Part model, mm, in its own coordinate system. A direction names the side the tool comes from. Give positions to 0.01 mm unless a question says otherwise; leave off trailing zeros. Write each loop counter-clockwise with the first axis right and the second up, starting at its lowest first coordinate (ties: lowest second). Pieces come first, ordered by that corner, then holes. Notation, with made-up numbers: M 44.25,45.5 L 69.25,45.5 A25 cw 69.25,72.5 Z; hole C -6,28.5 d11. An arc over 180 degrees is marked long. Use a Markdown table: item, result.
```python
from build123d import *

# Parameters (mm, degrees)
SKETCH1_W           = 71.12
SKETCH1_H           = 71.12
SKETCH1_R           = 1.905
BOSS_EXTRUDE1_DEPTH = 2.54
SKETCH2_R           = 2.54
SKETCH2_R_2         = 18.415
CUT_EXTRUDE1_DEPTH  = 3.54
SKETCH3_R           = 4.445
SKETCH3_R_2         = 1.905
BOSS_EXTRUDE2_DEPTH = 13.208
FILLET1_R           = 10.16


with BuildPart() as part:
    # Sketch1 → Boss-Extrude1 (new body)
    with BuildSketch(Plane(origin=(0, 0, 0), x_dir=(1, 0, 0), z_dir=(0, 1, 0))):
        with Locations((35.56, 35.56)):
            Rectangle(SKETCH1_W, SKETCH1_H)
        with Locations((8.5598, 62.5475)):
            Circle(SKETCH1_R, mode=Mode.SUBTRACT)
        with Locations((62.5475, 62.5602)):
            Circle(SKETCH1_R, mode=Mode.SUBTRACT)
        with Locations((62.5602, 8.5725)):
            Circle(SKETCH1_R, mode=Mode.SUBTRACT)
        with Locations((8.5725, 8.5598)):
            Circle(SKETCH1_R, mode=Mode.SUBTRACT)
    extrude(amount=BOSS_EXTRUDE1_DEPTH)

    # Sketch2 → Cut-Extrude1 (cut, through all)
    with BuildSketch(Plane(origin=(0, 2.54, 0), x_dir=(1, 0, 0), z_dir=(0, 1, 0))):
        with Locations((25.179834649, 12.479834649)):
            Circle(SKETCH2_R)
        with Locations((66.04, 53.34)):
            Circle(SKETCH2_R)
        with Locations((47.181462146, 34.481462146)):
            Circle(SKETCH2_R_2)
    extrude(amount=-CUT_EXTRUDE1_DEPTH, mode=Mode.SUBTRACT)

    # Sketch3 → Boss-Extrude2 (add)
    with BuildSketch(Plane.XZ):
        with Locations((62.5602, -8.5725)):
            Circle(SKETCH3_R)
        with Locations((62.5602, -8.5725)):
            Circle(SKETCH3_R_2, mode=Mode.SUBTRACT)
        with Locations((62.5475, -62.5602)):
            Circle(SKETCH3_R)
        with Locations((62.5475, -62.5602)):
            Circle(SKETCH3_R_2, mode=Mode.SUBTRACT)
        with Locations((8.5598, -62.5475)):
            Circle(SKETCH3_R)
        with Locations((8.5598, -62.5475)):
            Circle(SKETCH3_R_2, mode=Mode.SUBTRACT)
        with Locations((8.5725, -8.5598)):
            Circle(SKETCH3_R)
        with Locations((8.5725, -8.5598)):
            Circle(SKETCH3_R_2, mode=Mode.SUBTRACT)
    extrude(amount=BOSS_EXTRUDE2_DEPTH)

    # Fillet1
    fillet1_edges = [part.edges().sort_by_distance(p)[0] for p in [
        (0, 1.27, -71.12),
        (71.12, 1.27, -71.12),
        (71.12, 1.27, 0),
        (0, 1.27, 0),
    ]]
    fillet(fillet1_edges, radius=FILLET1_R)


solid = part.part
```
1. Cut at C-C, the plane z = -25. Give the cut face in (x, y), then the cut area to 3 significant figures.
Findings below:
| item | result |
|---|---|
| outline | M 0,0 L 31.39,0 L 31.39,2.54 L 0,2.54 Z; M 62.97,0 L 71.12,0 L 71.12,2.54 L 62.97,2.54 Z |
| area | 100 mm2 |
2. Tool access for faces 4 (the cylindrical face through (68.463, 1.288, -54.103)), 5 (the cylindrical face through (58.12, -6.51, -8.38)): list every direction of +Z, -Z, +X, -X, +Y, -Y with a clear straight run to the whole face (end or side of a thin tool).
Findings below:
| item | result |
|---|---|
| face 4 | +Y, -Y |
| face 5 | -Y |
3. Drop flat-ended pins along their axis: P1, Ø1.5, axis at y = -11.5, z = -12, coming from the +X side; P2, Ø8, axis at x = 10, y = -9, coming from the +Z side; P3, Ø4, axis at x = 29.5, z = -12, coming from the -Y side; P4, Ø3.5, axis at x = 62.56, z = -8.57, coming from the +Y side (3 decimals). Give the stop position or say it passes through.
Findings below:
| item | result |
|---|---|
| P1 | x = 66.11 |
| P2 | z = -4.11 |
| P3 | y = 0 |
| P4 | through |
4. Two-plate mould, pull along Z, no slides. Class faces 1 (the cylindrical face through (7.596, -6.512, -66.887)), 2 (the cylindrical face through (68.223, 1.288, -3.055)), 3 (the flat face through (9.5, -13.208, -10.5)): released by +Z, released by -Z, zero draft, split by the parting line, or undercut.
Findings below:
| item | result |
|---|---|
| face 1 | undercut |
| face 2 | released by +Z |
| face 3 | zero draft |
5. Cut at B-B, the plane x = 32. Give the cut face in (y, z), then the cut area to 3 significant figures.
Findings below:
| item | result |
|---|---|
| outline | M 0,-71.12 L 2.54,-71.12 L 2.54,-44.9 L 0,-44.9 Z; M 0,-24.06 L 2.54,-24.06 L 2.54,0 L 0,0 Z |
| area | 128 mm2 |
6. Cut at A-A, the plane y = -7.5. Give the cut face in (x, z) (1 decimal).
Findings below:
| item | result |
|---|---|
| outline | C 8.6,-62.5 d8.9; C 8.6,-8.6 d8.9; C 62.5,-62.6 d8.9; C 62.6,-8.6 d8.9; hole C 8.6,-62.5 d3.8; hole C 8.6,-8.6 d3.8; hole C 62.5,-62.6 d3.8; hole C 62.6,-8.6 d3.8 |
7. Cut at D-D, the plane z = -5. Give the cut face in (x, y), then the cut area to 3 significant figures.
Findings below:
| item | result |
|---|---|
| outline | M 1.41,0 L 5.91,0 L 5.91,-13.21 L 11.23,-13.21 L 11.23,0 L 59.92,0 L 59.92,-13.21 L 65.21,-13.21 L 65.21,0 L 69.71,0 L 69.71,2.54 L 1.41,2.54 Z |
| area | 314 mm2 |
8. Drill centre lines: L1, parallel to X at y = 1.25, z = -53.5; L2, parallel to X at y = -5, z = -9; L3, parallel to Y at x = 19, z = -24.5. Where is each one in solid material? Low to high.
Findings below:
| item | result |
|---|---|
| L1 | 0 to 63.51, 68.57 to 71.12 |
| L2 | 4.15 to 6.72, 10.43 to 13, 58.14 to 60.7, 64.42 to 66.98 |
| L3 | 0 to 2.54 |
